Geometry check sheet. Reference: the model listing, model coordinates, mm. Face numbers are marked on the shaded views. A direction names the side the tool comes from. Give positions to 0.01 mm unless a question says otherwise; leave off trailing zeros. Order: outer loops, then holes, each group sorted by start corner. A loop starts at its lowest first (then second) coordinate and runs counter-clockwise, first axis right, second up. Notation, with made-up numbers: M -35.75,5 L 18.25,5 A16 ccw 18.25,20 Z; hole C 82,16.5 d9. An arc over 180 degrees is marked long. Use CSV: the item, a comma, the result in double quotes. Start each with the question number.
from build123d import *

# Parameters (mm, degrees)
F0_R            = 25
F1_DEPTH        = 125
F3_DEPTH        = 5
F3_COPIES_COUNT = 4


# Not quite as in the source:
# - a pattern or mirror of a feature is missing from the dataset's text; its kind, count and spacing are read off the source's solid


with BuildPart() as f1:
    # F0 (on Top) → F1 (new body)
    with BuildSketch(Plane.XY):
        Circle(F0_R)
    extrude(amount=F1_DEPTH)

    # F2 (on Front) → F3 (join, symmetric)
    with BuildSketch(Plane.XZ):
        Polygon((0, 60), (0, 0), (60, 0), align=None)
    f3 = extrude(amount=F3_DEPTH, both=True)

    # F3_copies: F3 ×4 about axis
    f3_copies_axis = Axis((0, 0, 0), (0, 0, 1))
    for i in range(1, F3_COPIES_COUNT):
        add(f3.rotate(f3_copies_axis, i * 360 / F3_COPIES_COUNT))

    # F4 (on Front) → F5 (revolve)
    with BuildSketch(Plane.XZ):
        Polygon((0, 156.9369882345), (-25.1428224146, 125.2296715975), (0, 124.8316764832), align=None)
    revolve(axis=Axis((0, 0, 140.8843323588), (0, 0, -1)))


solid = f1.part
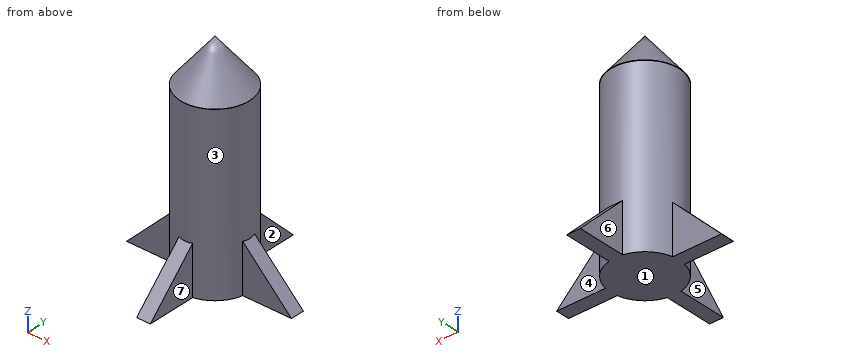
(1) Access from +Z, -Z, +X, -X, +Y, -Y to the whole of each face (thin tool, end or side, straight path). Record for the marked faces 4, 5, 6 and 7.
(2) Sectioned sample at B-B on y = 41.5. Record the cut outline in (x, z).
(3) Sectioned sample at C-C on z = 41. Record the cut outline in (x, y).
(4) Thickness scan on line 1 (X direction, y = 28, z = 20); line 2 (Z direction, x = 21, y = -3); line 3 (Y direction, x = -19, z = 8). Record the ranges inside material, lowest first.
(5) Sectioned sample at D-D on z = 147. Record the cut outline in (x, y), then the cut area to 3 significant figures.
(6) Draft check along Z on the marked faces 1, 2 and 3. Enter one of: +Z half, -Z half, draft (parallel to the pull), parting line (faces both ways), or undercut.
(7) Sectioned sample at A-A on x = -50. Record the cut outline in (y, z).
(8) Go/stop test with flat-tipped pins: P1, Ø2, axis at x = 2, z = 95.5, coming from the -Y side; P2, Ø18, axis at x = 39.5, z = 26, coming from the -Y side; P3, Ø1, axis at x = 9, z = 39, coming from the -Y side; P4, Ø10, axis at y = -42.5, z = 30.5, coming from the +X side. Record where each tip stops, or that it passes through.
Responses:
1,face 4,"+Z, -Z, +X, +Y"
1,face 5,"+Z, -Z, -X, -Y"
1,face 6,"+Z, -Z, -X, +Y"
1,face 7,"+Z, -Z, +X, -Y"
2,outline,"M -5,0 L 5,0 L 5,18.5 L -5,18.5 Z"
3,outline,"C 0,0 d50"
4,line 1,"-5 to 5"
4,line 2,"0 to 125, 125.17 to 130.19"
4,line 3,"-16.25 to 16.25"
5,outline,"C 0,0 d15.76"
5,area,"195 mm2"
6,face 1,"-Z half"
6,face 2,"draft"
6,face 3,"undercut"
7,outline,"M -5,0 L 5,0 L 5,10 L -5,10 Z"
8,P1,"y = -24.98"
8,P2,"y = -5"
8,P3,"y = -23.51"
8,P4,"through"
